Part model, mm, in its own coordinate system. A direction names the side the tool comes from. Round coordinates to 2 decimals unless told otherwise and drop trailing zeros. Loops run counter-clockwise (first coordinate to the right, second up) from the corner with the lowest first, then second, coordinate; pieces in that order, holes last.
1) Probe line 1 (Z direction, x = 7, y = 4.75); line 2 (X direction, y = 2.5, z = 17.5); line 3 (Z direction, x = 5.5, y = 0.25). List the from-to ranges inside material, lowest first.
2) Band-saw the part on B-B, the plane y = 2.5. Write the cut outline in (x, z).
3) Band-saw the part on D-D, the plane z = 39.5. Write the cut outline in (x, y), then the cut area to 3 significant figures.
4) 3-axis set-ups, long thin cutter, end or side, ignore diameter. For faces 1 (the flat face through (4, 1.5, 11)), 2 (the flat face through (-7, -2.6, 50)), 3 (the flat face through (0, 4.4, 36)), 4 (the flat face through (5, 3.903, 29)), 5 (the flat face through (9.3, 5, 50)): which of +Z, -Z, +X, -X, +Y, -Y reach the whole face in a straight line?
5) Mould opens along X. For faces 6 (the cylindrical face through (0, -8, 27)), 7 (the flat face through (-5, 3.903, 43)), 8 (the flat face through (-8, 2, 17)), 9 (the flat face through (6, 1, 29)) say: +X half, -X half, draft (parallel to the pull), parting line (faces both ways), or undercut.
6) Band-saw the part on C-C, the plane x = 0. Write the cut outline in (y, z), then the cut area to 3 significant figures.
7) Drop flat-ended pins along their axis: P1, Ø2, axis at y = -0.5, z = 19, coming from the -X side; P2, Ø2, axis at y = -6, z = 5.5, coming from the -X side (3 decimals); P3, Ø1.9, axis at x = -4.5, z = 42, coming from the -Y side. Give the stop position or say it passes through.
8) Band-saw the part on A-A, the plane z = 49. Write the cut outline in (x, y), then the cut area to 3 significant figures.
from build123d import *

# Parameters (mm, degrees)
BOX005_W     = 3
BOX005_H     = 10
BOX005_DEPTH = 4
BOX004_W     = 3
BOX004_H     = 10
BOX004_DEPTH = 4
BOX003_W     = 3
BOX003_H     = 10
BOX003_DEPTH = 4
BOX002_W     = 3
BOX002_H     = 10
BOX002_DEPTH = 4
BOX001_W     = 18.4
BOX001_H     = 7
BOX001_DEPTH = 4
BOX_W        = 18.4
BOX_H        = 7
BOX_DEPTH    = 4
PAD001_DEPTH = 34
PAD_DEPTH    = 55


with BuildPart() as obj1:
    # Box005 → Box005 (new body)
    with BuildSketch(Plane(origin=(6.3, -2.6, 34.2), x_dir=(1, 0, 0), z_dir=(0, 0, 1))):
        with Locations((1.5, 5)):
            Rectangle(BOX005_W, BOX005_H)
    extrude(amount=BOX005_DEPTH)


with BuildPart() as obj2:
    # Box004 → Box004 (new body)
    with BuildSketch(Plane(origin=(-9.1, -2.6, 34.2), x_dir=(1, 0, 0), z_dir=(0, 0, 1))):
        with Locations((1.5, 5)):
            Rectangle(BOX004_W, BOX004_H)
    extrude(amount=BOX004_DEPTH)


with BuildPart() as obj3:
    # Box003 → Box003 (new body)
    with BuildSketch(Plane(origin=(6.3, -2.6, 48.2), x_dir=(1, 0, 0), z_dir=(0, 0, 1))):
        with Locations((1.5, 5)):
            Rectangle(BOX003_W, BOX003_H)
    extrude(amount=BOX003_DEPTH)


with BuildPart() as obj4:
    # Box002 → Box002 (new body)
    with BuildSketch(Plane(origin=(-9.1, -2.6, 48.2), x_dir=(1, 0, 0), z_dir=(0, 0, 1))):
        with Locations((1.5, 5)):
            Rectangle(BOX002_W, BOX002_H)
    extrude(amount=BOX002_DEPTH)


with BuildPart() as obj5:
    # Box001 → Box001 (new body)
    with BuildSketch(Plane(origin=(-9.1, -2.6, 34.2), x_dir=(1, 0, 0), z_dir=(0, 0, 1))):
        with Locations((9.2, 3.5)):
            Rectangle(BOX001_W, BOX001_H)
    extrude(amount=BOX001_DEPTH)


with BuildPart() as obj6:
    # Box → Box (new body)
    with BuildSketch(Plane(origin=(-9.1, -2.6, 48.2), x_dir=(1, 0, 0), z_dir=(0, 0, 1))):
        with Locations((9.2, 3.5)):
            Rectangle(BOX_W, BOX_H)
    extrude(amount=BOX_DEPTH)


with BuildPart() as kegel:
    # Cone → Cone (revolve)
    with BuildSketch(Plane(origin=(0, -7.3, 5.7), x_dir=(1, 0, 0), z_dir=(0, -1, 0))):
        Polygon((0, 0), (5, 0), (4, 12), (0, 12), align=None)
    revolve(axis=Axis((0, -7.3, 5.7), (0, 0, 1)))


with BuildPart() as body001:
    # Sketch001 → Pad001 (new body)
    with BuildSketch(Plane.XY):
        with BuildLine():
            Line((-6, -0.697355), (-6, 4.302645))
            Line((-6, 4.302645), (6, 4.302645))
            Line((6, 4.302645), (6, -0.697355))
            ThreePointArc((-6, -0.697355), (0, -6.040389), (6, -0.697355))
        make_face()
    extrude(amount=PAD001_DEPTH)


with BuildPart() as body001_1:
    # Body001 placement: moved
    add(body001.part.moved(Location((0, -0.4, 23.3))))


with BuildPart() as cut007:
    # Sketch → Pad (new body)
    with BuildSketch(Plane.XY):
        with BuildLine():
            ThreePointArc((-8, 0), (0, -8), (8, 0))
            Line((8, 4), (8, 0))
            Line((10, 4), (8, 4))
            Line((10, 5.5), (10, 4))
            Line((-10, 5.5), (10, 5.5))
            Line((-10, 4), (-10, 5.5))
            Line((-8, 4), (-10, 4))
            Line((-8, 0), (-8, 4))
        make_face()
        with BuildLine():
            ThreePointArc((-3.65, -1), (0, -3.784508), (3.65, -1))
            Line((3.65, -1), (5, -1))
            Line((5, 1.5), (5, -1))
            Line((3.65, 1.5), (5, 1.5))
            Line((3.65, 4), (3.65, 1.5))
            Line((-3.65, 4), (3.65, 4))
            Line((-3.65, 1.5), (-3.65, 4))
            Line((-3.65, 1.5), (-5, 1.5))
            Line((-5, 1.5), (-5, -1))
            Line((-3.65, -1), (-5, -1))
        make_face(mode=Mode.SUBTRACT)
    extrude(amount=PAD_DEPTH)

    # Cut: cut Body001
    add(body001_1.part, mode=Mode.SUBTRACT)

    # Cut001: cut Kegel
    add(kegel.part, mode=Mode.SUBTRACT)

    # Cut002: cut obj6
    add(obj6.part, mode=Mode.SUBTRACT)

    # Cut003: cut obj5
    add(obj5.part, mode=Mode.SUBTRACT)

    # Cut004: cut obj4
    add(obj4.part, mode=Mode.SUBTRACT)

    # Cut005: cut obj3
    add(obj3.part, mode=Mode.SUBTRACT)

    # Cut006: cut obj2
    add(obj2.part, mode=Mode.SUBTRACT)

    # Cut007: cut obj1
    add(obj1.part, mode=Mode.SUBTRACT)


solid = cut007.part
Reported:
1. line 1: z = 0 to 34.2, 38.2 to 48.2, 52.2 to 55
1. line 2: x = -8 to -3.65, 3.65 to 8
1. line 3: z = 0 to 23.3
2. outline: (-8, 0) - (-3.65, 0) - (-3.65, 23.3) - (-6, 23.3) - (-6, 34.2) - (-8, 34.2) - close; (-8, 38.2) - (-6, 38.2) - (-6, 48.2) - (-8, 48.2) - close; (-8, 52.2) - (-6, 52.2) - (-6, 55) - (-8, 55) - close; (3.65, 0) - (8, 0) - (8, 34.2) - (6, 34.2) - (6, 23.3) - (3.65, 23.3) - close; (6, 38.2) - (8, 38.2) - (8, 48.2) - (6, 48.2) - close; (6, 52.2) - (8, 52.2) - (8, 55) - (6, 55) - close
3. outline: (-10, 4) - (-8, 4) - (-8, 0) arc R8 ccw to (8, 0) - (8, 4) - (10, 4) - (10, 5.5) - (-10, 5.5) - close; hole (-6, -1.1) arc R6.04 ccw to (6, -1.1) - (6, 3.9) - (3.65, 3.9) - (3.65, 4) - (-3.65, 4) - (-3.65, 3.9) - (-6, 3.9) - close
3. area: 84.9 mm2
4. face 1: +Z, -Z
4. face 2: +X, -X
4. face 3: none
4. face 4: +Z
4. face 5: +Y, -Y
5. face 6: parting line
5. face 7: undercut
5. face 8: -X half
5. face 9: undercut
6. outline: (-8, 0) - (-3.78, 0) - (-3.78, 5.7) - (-8, 5.7) - close; (-8, 17.7) - (-3.78, 17.7) - (-3.78, 23.3) - (-6.44, 23.3) - (-6.44, 55) - (-8, 55) - close; (4, 0) - (5.5, 0) - (5.5, 55) - (4, 55) - (4, 52.2) - (4.4, 52.2) - (4.4, 48.2) - (4, 48.2) - (4, 38.2) - (4.4, 38.2) - (4.4, 34.2) - (4, 34.2) - close
6. area: 176 mm2
7. P1: stops at x = -8
7. P2: stops at x = -6.245
7. P3: stops at y = -7.17
8. outline: (-10, 4) - (-9.1, 4) - (-9.1, 5.5) - (-10, 5.5) - close; (-7.57, -2.6) arc R8 ccw to (7.57, -2.6) - (5.63, -2.6) arc R6.04 cw to (-5.63, -2.6) - close; (-6.1, 4.4) - (6.3, 4.4) - (6.3, 5.5) - (-6.1, 5.5) - close; (9.3, 4) - (10, 4) - (10, 5.5) - (9.3, 5.5) - close
8. area: 44.4 mm2
